```python
from build123d import *

# Parameters (mm, degrees)
SKETCH_W        = 72
SKETCH_H        = 72
PAD_DEPTH       = 1.5
PAD001_DEPTH    = 4
SKETCH002_R     = 1.6
POCKET_DEPTH    = 5.501
SKETCH003_W     = 11
SKETCH003_H     = 41
SKETCH003_W_2   = 13
SKETCH003_H_2   = 36
SKETCH003_W_3   = 9
SKETCH003_H_3   = 9
PAD002_DEPTH    = 4
FILLET_R        = 2
CHAMFER_SIZE    = 1
FILLET001_R     = 2
CHAMFER001_SIZE = 1


with BuildPart() as part:
    # Sketch → Pad (new body)
    with BuildSketch(Plane.XY):
        with Locations((36, -36)):
            Rectangle(SKETCH_W, SKETCH_H)
    extrude(amount=PAD_DEPTH)

    # Sketch001 (on Face6 of Pad) → Pad001 (join)
    with BuildSketch(Plane.XY.offset(1.5)):
        with BuildLine():
            ThreePointArc((0, -8), (5.656854, -5.656854), (8, 0))
            Line((0, 0), (8, 0))
            Line((0, -8), (0, 0))
        make_face()
        with BuildLine():
            ThreePointArc((8, -72), (5.656854, -66.343146), (0, -64))
            Line((0, -72), (0, -64))
            Line((8, -72), (0, -72))
        make_face()
        with BuildLine():
            ThreePointArc((72, -64), (66.343146, -66.343146), (64, -72))
            Line((64, -72), (72, -72))
            Line((72, -72), (72, -64))
        make_face()
        with BuildLine():
            ThreePointArc((64, 0), (66.343146, -5.656854), (72, -8))
            Line((72, -8), (72, 0))
            Line((72, 0), (64, 0))
        make_face()
    extrude(amount=PAD001_DEPTH)

    # Sketch002 (on Face14 of Pad001) → Pocket (cut, through all)
    with BuildSketch(Plane.XY.offset(5.5)):
        with Locations((4, -4)):
            Circle(SKETCH002_R)
        with Locations((68, -4)):
            Circle(SKETCH002_R)
        with Locations((68, -68)):
            Circle(SKETCH002_R)
        with Locations((4, -68)):
            Circle(SKETCH002_R)
    extrude(amount=-POCKET_DEPTH, mode=Mode.SUBTRACT)

    # Sketch003 (on Face6 of Pocket) → Pad002 (join)
    with BuildSketch(Plane.XY.offset(1.5)):
        with Locations((25.5, -47.5)):
            Rectangle(SKETCH003_W, SKETCH003_H)
        with Locations((47.5, -50)):
            Rectangle(SKETCH003_W_2, SKETCH003_H_2)
        with Locations((48.5, -16.5)):
            Rectangle(SKETCH003_W_3, SKETCH003_H_3)
    extrude(amount=PAD002_DEPTH)

    # Fillet
    fillet_edges = [part.edges().sort_by_distance(p)[0] for p in [
        (20, -68, 3.5),
        (31, -68, 3.5),
        (31, -27, 3.5),
        (20, -27, 3.5),
        (44, -12, 3.5),
        (53, -12, 3.5),
        (53, -21, 3.5),
        (44, -21, 3.5),
        (41, -32, 3.5),
        (54, -32, 3.5),
        (54, -68, 3.5),
        (41, -68, 3.5),
    ]]
    fillet(fillet_edges, radius=FILLET_R)

    # Chamfer
    chamfer_edges = [part.edges().sort_by_distance(p)[0] for p in [
        (20, -47.5, 5.5),
        (41, -50, 5.5),
        (44, -16.5, 5.5),
    ]]
    chamfer(chamfer_edges, length=CHAMFER_SIZE)

    # Fillet001
    fillet001_edges = [part.edges().sort_by_distance(p)[0] for p in [
        (72, -72, 3.5),
        (0, -72, 3.5),
        (0, 0, 3.5),
        (72, 0, 3.5),
    ]]
    fillet(fillet001_edges, radius=FILLET001_R)

    # Chamfer001
    chamfer001_edges = [part.edges().sort_by_distance(p)[0] for p in [
        (72, -36, 0),
    ]]
    chamfer(chamfer001_edges, length=CHAMFER001_SIZE)


solid = part.part
```
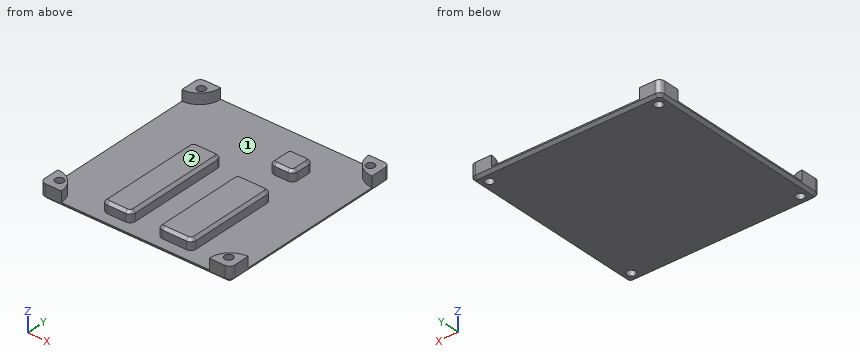
Read the model definition and answer for the solid it produces. Units are mm, in the model's axes. Face numbers are marked on the shaded views. Coordinates: 2 decimals unless noted, no trailing zeros. Order: outer loops, then holes, each group sorted by start corner. A loop starts at its lowest first (then second) coordinate and runs counter-clockwise, first axis right, second up. Notation, with made-up numbers: (84.25, -21) - (129.25, -21) arc R18 cw to (129.25, -16) - close; hole circle Ø6 at (-27, 34.5). An arc over 180 degrees is marked (long way). Answer as a JSON object with one key per item and string values. Group by question number.
Item 1: Section A-A (z = 3.45) is taken. State how many separate pieces and enclosed holes the cut face has, plus the area to 3 significant figures.
Item 2: Flat-ended cylindrical pins translate along their axes: P1, Ø1.5, axis at x = 49.5, z = 3.5, coming from the -Y side; P2, Ø1.5, axis at y = -17.5, z = 2.5, coming from the +X side; P3, Ø2.5, axis at y = -55, z = 3.5, coming from the +X side. Find the tip coordinate at first contact, or state that the pin passes through.
Item 3: The mould has two halves that part along Y. Classify the marked faces 1 and 2: +Y half, -Y half, draft (parallel to the pull), parting line (faces both ways), or undercut.
Item 4: Section C-C (y = -4) is taken. Give the vertices of the cut face in (x, z), plus the area to 3 significant figures.
Item 5: Section B-B (y = -17) is taken. Give the vertices of the cut face in (x, z), plus the area to 3 significant figures.
Item 6: Section D-D (x = 12) is taken. Give the vertices of the cut face in (y, z).
Item 7: Consider probe 1 along Y at (x, z) = (68, 3.25); probe 2 along X at (y, z) = (-48, 2.5); probe 3 along Y at (x, z) = (46, 2). Determine where each line is inside the solid, lowest interval first. Write a range as from..to.
Results are:
{
 "1": {"separate pieces": "7", "enclosed holes": "4", "area": "1,160 mm^2"},
 "2": {"P1": "stops at y = -68", "P2": "stops at x = 53", "P3": "stops at x = 54"},
 "3": {"face 1": "undercut", "face 2": "draft"},
 "4": {"outline": "(0, 1) - (1, 0) - (2.4, 0) - (2.4, 5.5) - (0, 5.5) - close; (5.6, 0) - (66.4, 0) - (66.4, 5.5) - (65.07, 5.5) - (65.07, 1.5) - (6.93, 1.5) - (6.93, 5.5) - (5.6, 5.5) - close; (69.6, 0) - (71, 0) - (72, 1) - (72, 5.5) - (69.6, 5.5) - close", "area": "127 mm^2"},
 "5": {"outline": "(0, 1) - (1, 0) - (71, 0) - (72, 1) - (72, 1.5) - (53, 1.5) - (53, 4.5) - (52, 5.5) - (45, 5.5) - (44, 4.5) - (44, 1.5) - (0, 1.5) - close", "area": "142 mm^2"},
 "6": {"outline": "(-72, 1) - (-71, 0) - (-1, 0) - (0, 1) - (0, 1.5) - (-72, 1.5) - close"},
 "7": {"probe 1": "y = -72..-69.6, -66.4..-65.07, -6.93..-5.6, -2.4..0", "probe 2": "x = 20..31, 41..54", "probe 3": "y = -68..-32, -21..-12"}
}
